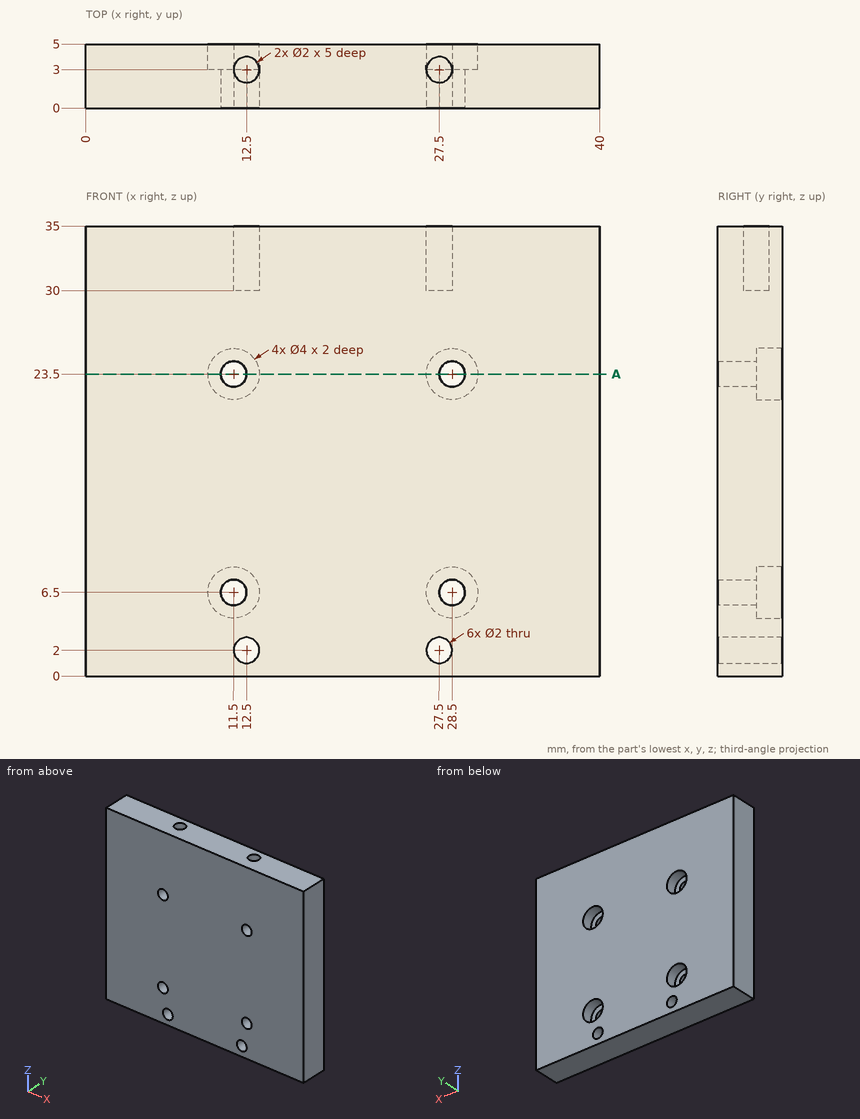
The figure shows three views and two pictorial views of one solid part (mm, origin at its lowest corner). Answer the questions. Give positions to 0.01 mm unless a question says otherwise; leave off trailing zeros. Loops run counter-clockwise (first coordinate to the right, second up) from the corner with the lowest first, then second, coordinate; pieces in that order, holes last. Notation, with made-up numbers: (16, 11.25) -> (40, 11.25) arc R18 ccw to (40, 30.25) -> close; hole circle Ø2 at (81.5, 71.5). An arc over 180 degrees is marked (long way). Use a Markdown table: item, result. Add a question column.
1. Find the intervals of material crossed by probe 1 along X at (y, z) = (3.75, 6.5); probe 2 along X at (y, z) = (1.8, 23.5); probe 3 along Z at (x, y) = (12, 0.95), in increasing order.
2. Flat-ended cylindrical pins translate along their axes: pin 1 Ø1.8 at (x, z) = (12.5, 2) entering from -Y; pin 2 Ø0.6 at (x, y) = (12.5, 3) entering from +Z; pin 3 Ø3 at (x, z) = (28.5, 23.5) entering from +Y. Find the tip coordinate at first contact, or state that the pin passes through.
3. Section A-A on z = 23.5 is taken. Determine the outline of the cut face in (x, y), and give its area (3 significant figures).
Results below:
| question | item | result |
|---|---|---|
| 1 | probe 1 | x = 0 to 9.5, 13.5 to 26.5, 30.5 to 40 |
| 1 | probe 2 | x = 0 to 10.5, 12.5 to 27.5, 29.5 to 40 |
| 1 | probe 3 | z = 0 to 1.13, 2.87 to 5.63, 7.37 to 22.63, 24.37 to 35 |
| 2 | pin 1 | passes through |
| 2 | pin 2 | stops at z = 30 |
| 2 | pin 3 | stops at y = 3 |
| 3 | outline | (0, 0) -> (10.5, 0) -> (10.5, 3) -> (9.5, 3) -> (9.5, 5) -> (0, 5) -> close; (12.5, 0) -> (27.5, 0) -> (27.5, 3) -> (26.5, 3) -> (26.5, 5) -> (13.5, 5) -> (13.5, 3) -> (12.5, 3) -> close; (29.5, 0) -> (40, 0) -> (40, 5) -> (30.5, 5) -> (30.5, 3) -> (29.5, 3) -> close |
| 3 | area | 172 mm^2 |
